```python
from build123d import *

# Parameters (mm, degrees)
F0_W     = 160.32
F0_H     = 134.37
F0_R     = 2.25
F1_DEPTH = 3.175


# Not quite as in the source:
# - a length typed as a fraction of an inch, garbled in the dataset ("3 / 203.2 mm" for 3/8 in), is restored


with BuildPart() as f1:
    # F0 (on Top) → F1 (new body)
    with BuildSketch(Plane.XY):
        with Locations((-15, 57.025)):
            Rectangle(F0_W, F0_H)
        with Locations((-65, 14.05)):
            Circle(F0_R, mode=Mode.SUBTRACT)
        with BuildLine():
            ThreePointArc((0, 2.25), (1.5909902577, 1.5909902577), (2.25, 0))
            ThreePointArc((2.25, 0), (-1.5909902577, -1.5909902577), (0, 2.25))
        make_face(mode=Mode.SUBTRACT)
        with Locations((35, 14.05)):
            Circle(F0_R, mode=Mode.SUBTRACT)
        with Locations((-85, 82.3)):
            Circle(F0_R, mode=Mode.SUBTRACT)
        with Locations((-65, 114.05)):
            Circle(F0_R, mode=Mode.SUBTRACT)
        with Locations((55, 82.3)):
            Circle(F0_R, mode=Mode.SUBTRACT)
        with Locations((35, 114.05)):
            Circle(F0_R, mode=Mode.SUBTRACT)
    extrude(amount=F1_DEPTH)


solid = f1.part
```
Input: part model. Units: mm. Frame: model coordinates. Give positions to 0.01 mm unless a question says otherwise; leave off trailing zeros. Write each loop counter-clockwise with the first axis right and the second up, starting at its lowest first coordinate (ties: lowest second). Pieces come first, ordered by that corner, then holes. Notation, with made-up numbers: (85.5, 24.25) - (138.5, 24.25) arc R14 ccw to (138.5, 35.25) - close; hole circle Ø1 at (50.25, 64.25). An arc over 180 degrees is marked (long way). Write item = value, one per line. Start each with the question number.
1. Mould query, pull axis Y, two halves, no side actions, for faces 1 (the flat face through (65.16, 56, 2)), 2 (the cylindrical face through (-66.66, 115.57, 1.57)), 3 (the flat face through (-16, -10.16, 2)). Classes: released by +Y, released by -Y, zero draft, split by the parting line, or undercut.
2. Ray query, L1, parallel to Y at x = 35, z = 0.7; L2, parallel to Y at x = -85, z = 1.35; L3, parallel to X at y = 12.5, z = 2.2. Return the intervals inside material, ascending.
3. Section query B-B, the plane y = 114.05. Output: boundary loops of the cut face in (x, z) (3 decimals), then the cut area to 3 significant figures.
4. Section query A-A, the plane x = 55. Output: boundary loops of the cut face in (y, z) (3 decimals), then the cut area to 3 significant figures.
5. First-contact query: pin 1 Ø5 at (x, y) = (55, 82.3) entering from +Z (3 decimals). Flat tip, straight axial feed; report the tip coordinate or a pass-through.
6. Section query C-C, the plane x = 35. Output: boundary loops of the cut face in (y, z) (3 decimals).
Check sheet entries:
q1.face_1 = zero draft
q1.face_2 = undercut
q1.face_3 = released by -Y
q2.L1 = -10.16 to 11.8, 16.3 to 111.8, 116.3 to 124.21
q2.L2 = -10.16 to 80.05, 84.55 to 124.21
q2.L3 = -95.16 to -66.63, -63.37 to 33.37, 36.63 to 65.16
q3.outline = (-95.16, 0) - (-67.25, 0) - (-67.25, 3.175) - (-95.16, 3.175) - close; (-62.75, 0) - (32.75, 0) - (32.75, 3.175) - (-62.75, 3.175) - close; (37.25, 0) - (65.16, 0) - (65.16, 3.175) - (37.25, 3.175) - close
q3.area = 480 mm2
q4.outline = (-10.16, 0) - (80.05, 0) - (80.05, 3.175) - (-10.16, 3.175) - close; (84.55, 0) - (124.21, 0) - (124.21, 3.175) - (84.55, 3.175) - close
q4.area = 412 mm2
q5.pin_1 = 3.175
q6.outline = (-10.16, 0) - (11.8, 0) - (11.8, 3.175) - (-10.16, 3.175) - close; (16.3, 0) - (111.8, 0) - (111.8, 3.175) - (16.3, 3.175) - close; (116.3, 0) - (124.21, 0) - (124.21, 3.175) - (116.3, 3.175) - close
